Design review of the part built by this model. Coordinates are the model's own, in mm. A direction names the side the tool comes from. Coordinates: 2 decimals unless noted, no trailing zeros. Loops run counter-clockwise (first coordinate to the right, second up) from the corner with the lowest first, then second, coordinate; pieces in that order, holes last. Notation, with made-up numbers: (17.25, 15) -> (43.25, 15) arc R23 ccw to (43.25, 51) -> close; hole circle Ø1 at (22, 87.25). An arc over 180 degrees is marked (long way). Use a Markdown table: item, result. Add a question column.
Q1. Take a section at B-B on y = 4. Write out the cut boundary in (x, z), plus the area to 3 significant figures.
Q2. Take a section at C-C on x = 20.5. Write out the cut boundary in (y, z), plus the area to 3 significant figures.
Q3. Take a section at A-A on z = 6. Write out the cut boundary in (x, y).
Q4. Draft analysis for pull direction Z (two halves, no side actions). For faces 1 (the face through (16.97, 5.12, -29.6)), 2 (the face through (17.901, 4.478, -30.795)), 3 (the face through (-34.12, 5, 0)), state which applies: pulls with the +Z half, pulls with the -Z half, needs draft (parallel to the pull), parting line crosses it, or undercut.
Q5. For probe 1 along Y at (x, z) = (13, 26); probe 2 along Z at (x, y) = (20, 3); probe 3 along Z at (x, y) = (15.5, 6.25), list the stretches that pass through material, from the lowest coordinate up.
Q6. Take a section at D-D on z = -19. Write out the cut boundary in (x, y).
Q7. For faces 4 (the face through (18, 6.1, 32)), 5 (the face through (-35, 5, 7.5)), 6 (the face through (-35, 5, -7.5)), 7 (the face through (-35.62, 4, 0)), 8 (the face through (17.151, 5.118, 29.496)), list the 3-axis set-ups (+Z, -Z, +X, -X, +Y, -Y) from which the entire face can be reached by the end or side of a thin tool; tool diameter is ignored.
Q8. Clearance check with flat-ended pins moving along their axes: pin 1 Ø2 at (y, z) = (5, -2) entering from +X; pin 2 Ø1 at (x, y) = (9.5, 2) entering from -Z; pin 3 Ø1.5 at (y, z) = (5, -2.5) entering from -X. State where each tip first meets the part, or that it passes through.
from build123d import *

# Parameters (mm, degrees)
RESSALTO_EXTRUS_O1_DEPTH  = 2.9
RESSALTO_EXTRUS_O8_DEPTH  = 4.5
ESBO_O11_W                = 15
ESBO_O11_H                = 1.3
RESSALTO_EXTRUS_O12_DEPTH = 1.5
ESBO_O15_W                = 15
ESBO_O15_H                = 1.3
RESSALTO_EXTRUS_O13_DEPTH = 1.5
ESBO_O16_W                = 15
ESBO_O16_H                = 1.3
RESSALTO_EXTRUS_O14_DEPTH = 1.5
CORTE_EXTRUS_O5_DEPTH     = 75.128633488
CORTE_EXTRUS_O8_DEPTH     = 75.128633488
CORTE_EXTRUS_O9_DEPTH     = 73.843490871


with BuildPart() as part:
    # Esboço1 → Ressalto-extrusão1 (new body)
    with BuildSketch(Plane(origin=(0, 0, 0), x_dir=(1, 0, 0), z_dir=(0, 1, 0))):
        Polygon((-43.62, 11.068078609), (-43.62, 25.184018742), (-12.224762753, 43.310067418), (0, 50.368037484), (31.395237247, 32.241988808), (43.62, 25.184018742), (43.62, -11.068078609), (43.62, -25.184018742), (12.224762753, -43.310067418), (0, -50.368037484), (-31.395237247, -32.241988808), (-43.62, -25.184018742), align=None)
    extrude(amount=RESSALTO_EXTRUS_O1_DEPTH)

    # Esboço4 → Ressalto-extrusão8 (add)
    with BuildSketch(Plane(origin=(0, 2.9, 0), x_dir=(1, 0, 0), z_dir=(0, 1, 0))):
        Polygon((-34.12, 0), (-34.12, 7.5), (-35.62, 7.5), (-35.62, -7.5), (-34.12, -7.5), align=None)
        Polygon((17.06, -29.548786777), (10.564809472, -33.298786777), (11.314809472, -34.597824883), (24.305190528, -27.097824883), (23.555190528, -25.798786777), align=None)
        Polygon((17.06, 29.548786777), (23.555190528, 25.798786777), (24.305190528, 27.097824883), (11.314809472, 34.597824883), (10.564809472, 33.298786777), align=None)
    extrude(amount=RESSALTO_EXTRUS_O8_DEPTH)

    # Esboço11 → Ressalto-extrusão12 (add)
    with BuildSketch(Plane.ZY.offset(35.62)):
        with Locations((0, 6.75)):
            Rectangle(ESBO_O11_W, ESBO_O11_H)
    extrude(amount=RESSALTO_EXTRUS_O12_DEPTH)

    # Esboço15 → Ressalto-extrusão13 (add)
    with BuildSketch(Plane(origin=(17.81, 0, 30.847824883), x_dir=(0.8660254037844386, 0, -0.5000000000000001), z_dir=(0.5000000000000001, 0, 0.8660254037844386))):
        with Locations((0, 6.75)):
            Rectangle(ESBO_O15_W, ESBO_O15_H)
    extrude(amount=RESSALTO_EXTRUS_O13_DEPTH)

    # Esboço16 → Ressalto-extrusão14 (add)
    with BuildSketch(Plane(origin=(17.81, 0, -30.847824883), x_dir=(-0.8660254037844386, 0, -0.5000000000000003), z_dir=(0.5000000000000003, 0, -0.8660254037844386))):
        with Locations((0, 6.75)):
            Rectangle(ESBO_O16_W, ESBO_O16_H)
    extrude(amount=RESSALTO_EXTRUS_O14_DEPTH)

    # Esboço17 → Corte-extrusão5 (cut, through all)
    with BuildSketch(Plane(origin=(-6.495190528, 0, 3.75), x_dir=(0.5000000000000064, 0, 0.866025403784435), z_dir=(-0.866025403784435, 0, 0.5000000000000064))):
        Polygon((35.62, 7.4), (37.12, 6.1), (38.522776478, 5.843708375), (38.659652416, 9.391906634), (36.37, 10.122640071), align=None)
    extrude(amount=-CORTE_EXTRUS_O5_DEPTH, mode=Mode.SUBTRACT)

    # Esboço18 → Corte-extrusão8 (cut, through all)
    with BuildSketch(Plane(origin=(6.495190528, 0, 3.75), x_dir=(0.5000000000000058, 0, -0.8660254037844354), z_dir=(0.8660254037844353, 0, 0.5000000000000057))):
        Polygon((35.62, 7.892314529), (37.556003767, 7.892314529), (38.139037221, 7.11493659), (37.685566756, 6.037944237), (37.12, 6.1), (35.62, 7.4), align=None)
    extrude(amount=-CORTE_EXTRUS_O8_DEPTH, mode=Mode.SUBTRACT)

    # Esboço19 → Corte-extrusão9 (cut, through all)
    with BuildSketch(Plane.XY.offset(7.5)):
        Polygon((-35.62, 8.416432615), (-35.62, 7.4), (-37.12, 6.1), (-37.526082167, 5.478521924), (-38.26778421, 5.863821686), (-38.576024021, 7.74215803), align=None)
    extrude(amount=-CORTE_EXTRUS_O9_DEPTH, mode=Mode.SUBTRACT)


solid = part.part
Answer list:
| question | item | result |
|---|---|---|
| 1 | outline | (-35.62, -7.5) -> (-34.12, -7.5) -> (-34.12, 7.5) -> (-35.62, 7.5) -> close; (10.56, -33.3) -> (11.31, -34.6) -> (24.31, -27.1) -> (23.56, -25.8) -> close; (10.56, 33.3) -> (23.56, 25.8) -> (24.31, 27.1) -> (11.31, 34.6) -> close |
| 1 | area | 67.5 mm² |
| 2 | outline | (0, -38.53) -> (2.9, -38.53) -> (2.9, -29.29) -> (6.1, -29.29) -> (6.1, -31.03) -> (7.4, -29.29) -> (7.4, -27.56) -> (2.9, -27.56) -> (2.9, 27.56) -> (7.4, 27.56) -> (7.4, 29.29) -> (6.1, 31.03) -> (6.1, 29.29) -> (2.9, 29.29) -> (2.9, 38.53) -> (0, 38.53) -> close |
| 2 | area | 241 mm² |
| 3 | outline | (-43.62, 0) -> (43.62, 0) -> (43.62, 2.9) -> (-34.12, 2.9) -> (-34.12, 7.4) -> (-35.62, 7.4) -> (-37.12, 6.1) -> (-35.62, 6.1) -> (-35.62, 2.9) -> (-43.62, 2.9) -> close |
| 4 | face 1 | undercut |
| 4 | face 2 | pulls with the -Z half |
| 4 | face 3 | needs draft |
| 5 | probe 1 | 0 to 2.9 |
| 5 | probe 2 | -29.58 to -27.85, 27.85 to 29.58 |
| 5 | probe 3 | -33.71 to -30.45, 30.45 to 33.71 |
| 6 | outline | (-43.62, 0) -> (43.62, 0) -> (43.62, 2.9) -> (-43.62, 2.9) -> close |
| 7 | face 4 | +Z, +X |
| 7 | face 5 | +Z, +X, -X, +Y |
| 7 | face 6 | -Z, +X, -X, +Y |
| 7 | face 7 | +Z, -Z, -X |
| 7 | face 8 | -X, +Y |
| 8 | pin 1 | x = -34.12 |
| 8 | pin 2 | z = -45.17 |
| 8 | pin 3 | x = -35.62 |
